The listing builds one solid part. Answer for the finished solid, in the listing's coordinates (mm). Round coordinates to 2 decimals unless told otherwise and drop trailing zeros. Write each loop counter-clockwise with the first axis right and the second up, starting at its lowest first coordinate (ties: lowest second). Pieces come first, ordered by that corner, then holes.
(1) A cutting plane is placed at A-A, the plane y = 0. Give the vertices of the cut face in (x, z), and give its area (3 significant figures).
(2) This flat-tipped pin is pushed along its axis until it touches: pin 1 Ø7.5 at (x, y) = (487.3, 0) entering from +Z. Where does it stop, or does it pass through?
(3) A cutting plane is placed at C-C, the plane z = 2.75. Give the vertices of the cut face in (x, y), and give its area (3 significant figures).
(4) Find the intervals of material crossed by probe 1 along Z at (x, y) = (327, 3); probe 2 along Y at (x, z) = (487.3, -12.5), in increasing order.
(5) A cutting plane is placed at D-D, the plane x = 12.7. Give the vertices of the cut face in (y, z), and give its area (3 significant figures).
(6) A cutting plane is placed at B-B, the plane x = 321.5. Give the vertices of the cut face in (y, z).
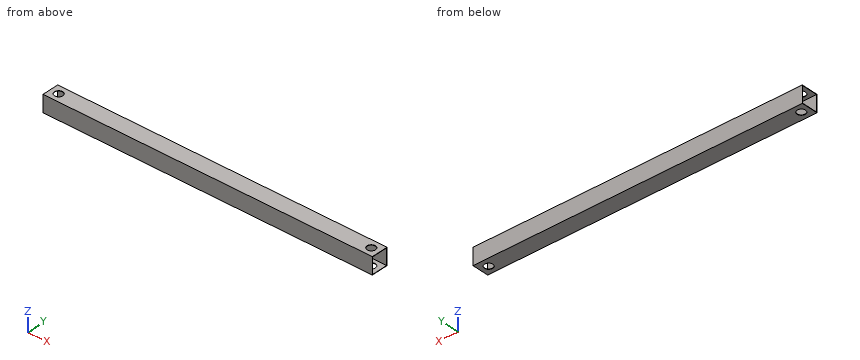
from build123d import *

# Parameters (mm, degrees)
SKETCH1_W                              = 25.4
SKETCH1_H                              = 25.4
SKETCH1_W_2                            = 24.2824
SKETCH1_H_2                            = 24.2824
AL_TUBE_SQUARE_1_SQ_X_022_WALL_3_DEPTH = 500
CROQUIS3_R                             = 6.35
CORTAR_EXTRUIR1_DEPTH                  = 501.805800685


with BuildPart() as part:
    # Sketch1 → Al tube (square) 1 SQ X .022 WALL(3) (new body)
    with BuildSketch(Plane.YZ):
        Rectangle(SKETCH1_W, SKETCH1_H)
        Rectangle(SKETCH1_W_2, SKETCH1_H_2, mode=Mode.SUBTRACT)
    extrude(amount=AL_TUBE_SQUARE_1_SQ_X_022_WALL_3_DEPTH)

    # Croquis3 → Cortar-Extruir1 (cut, through all)
    with BuildSketch(Plane.XY.offset(12.7)):
        with Locations((12.7, 0)):
            Circle(CROQUIS3_R)
        with Locations((487.3, 0)):
            Circle(CROQUIS3_R)
    extrude(amount=-CORTAR_EXTRUIR1_DEPTH, mode=Mode.SUBTRACT)


solid = part.part
Solutions:
1. outline: (0, -12.7) - (6.35, -12.7) - (6.35, -12.14) - (0, -12.14) - close; (0, 12.14) - (6.35, 12.14) - (6.35, 12.7) - (0, 12.7) - close; (19.05, -12.7) - (480.95, -12.7) - (480.95, -12.14) - (19.05, -12.14) - close; (19.05, 12.14) - (480.95, 12.14) - (480.95, 12.7) - (19.05, 12.7) - close; (493.65, -12.7) - (500, -12.7) - (500, -12.14) - (493.65, -12.14) - close; (493.65, 12.14) - (500, 12.14) - (500, 12.7) - (493.65, 12.7) - close
1. area: 530 mm2
2. pin 1: passes through
3. outline: (0, -12.7) - (500, -12.7) - (500, -12.14) - (0, -12.14) - close; (0, 12.14) - (500, 12.14) - (500, 12.7) - (0, 12.7) - close
3. area: 559 mm2
4. probe 1: z = -12.7 to -12.14, 12.14 to 12.7
4. probe 2: y = -12.7 to -6.35, 6.35 to 12.7
5. outline: (-12.7, -12.7) - (-6.35, -12.7) - (-6.35, -12.14) - (-12.14, -12.14) - (-12.14, 12.14) - (-6.35, 12.14) - (-6.35, 12.7) - (-12.7, 12.7) - close; (6.35, -12.7) - (12.7, -12.7) - (12.7, 12.7) - (6.35, 12.7) - (6.35, 12.14) - (12.14, 12.14) - (12.14, -12.14) - (6.35, -12.14) - close
5. area: 41.3 mm2
6. outline: (-12.7, -12.7) - (12.7, -12.7) - (12.7, 12.7) - (-12.7, 12.7) - close; hole (-12.14, -12.14) - (12.14, -12.14) - (12.14, 12.14) - (-12.14, 12.14) - close
